Could you check a few things on this model? Use its own coordinates, in mm. Face numbers are marked on the shaded views. A direction names the side the tool comes from. Coordinates: 2 decimals unless noted, no trailing zeros. Write each loop counter-clockwise with the first axis right and the second up, starting at its lowest first coordinate (ties: lowest second). Pieces come first, ordered by that corner, then holes.
Item 1: Which directions (+Z, -Z, +X, -X, +Y, -Y) give clear straight access to the entire face, cutting with the end or side of a thin tool? Please do the marked faces 1, 2 and 3.
Item 2: For P1, Ø2, axis at y = -48, z = 42.5, coming from the -X side; P2, Ø12, axis at x = 35, z = 8, coming from the -Y side; P3, Ø3, axis at x = 10, z = 10, coming from the -Y side, each with a flat end and sliding along its axis, tell me the tip position at first contact or that it passes through.
Item 3: I want a section at B-B on x = -21. Please give me the cut outline in (y, z), then the cut area to 3 significant figures.
Item 4: I want a section at A-A on z = -2.5. Please give me the cut outline in (x, y).
Item 5: Thinking about a two-plate mould opening in X: for the marked faces 4, 5 and 6, which applies, +X half, -X half, draft (parallel to the pull), parting line (faces both ways), or undercut?
Item 6: I want a section at D-D on z = 5. Please give me the cut outline in (x, y), then the cut area to 3 significant figures.
Item 7: I want a section at C-C on z = 47.5. Please give me the cut outline in (x, y), then the cut area to 3 significant figures.
Item 8: If I drill on probe 1 along Z at (x, y) = (57, -18.5); probe 2 along Y at (x, z) = (-22, 42.5); probe 3 along Z at (x, y) = (4.5, -5), over which ranges is the centre line in solid material (lowest first)?
from build123d import *

# Parameters (mm, degrees)
F1_DEPTH = 60
F3_DEPTH = 60.001
F5_DEPTH = 100.001


with BuildPart() as f1:
    # F0 (on Front) → F1 (new body)
    with BuildSketch(Plane.XZ):
        Polygon((68.4196182877, 52.7130502019), (-31.5803817123, 52.7130502019), (-31.5803817123, -7.2869497981), (-11.5803817123, -7.2869497981), (-11.5803817123, 7.7130502019), (23.4196182877, 7.7130502019), (23.4196182877, -7.2869497981), (38.4196182877, -7.2869497981), (38.4196182877, 12.7130502019), (68.4196182877, 12.7130502019), align=None)
    extrude(amount=F1_DEPTH)

    # F2 (on face) → F3 (cut, through all)
    with BuildSketch(Plane(origin=(0, 0, -7.2869497981), x_dir=(1, 0, 0), z_dir=(0, 0, -1))):
        Polygon((68.4196182877, 60), (43.4196182877, 60), (68.4196182877, 35), align=None)
        Polygon((18.4196182877, 60), (-31.5803817123, 60), (-31.5803817123, 40), (-16.2213978636, 40), align=None)
    extrude(amount=-F3_DEPTH, mode=Mode.SUBTRACT)

    # F4 (on face) → F5 (cut, through all)
    with BuildSketch(Plane.YZ.offset(68.4196182877)):
        Polygon((-60, 42.7130502019), (-60, -7.2869497981), (-5, -7.2869497981), (-27, 12.7130502019), (-35, 12.7130502019), (-35, 19.9857774746), align=None)
        Polygon((-35, 12.7130502019), (-27, 12.7130502019), (-35, 19.9857774746), align=None)
    extrude(amount=-F5_DEPTH, mode=Mode.SUBTRACT)


solid = f1.part
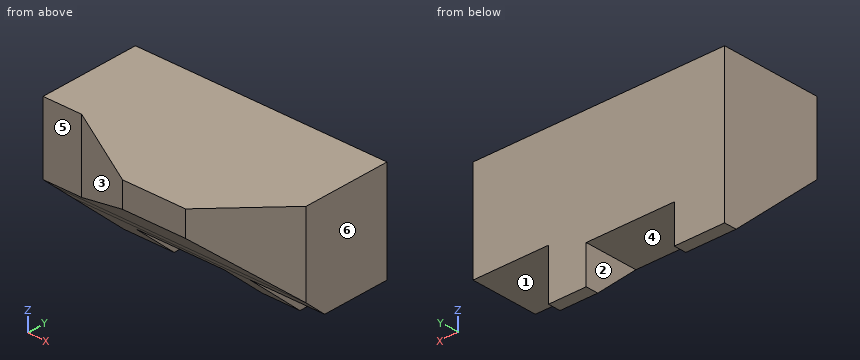
Response values:
1. face 1: -Z, +X, +Y, -Y
1. face 2: -Z, +Y, -Y
1. face 3: +Z, -Z, -X, -Y
2. P1: stops at x = -4.1
2. P2: stops at y = -28.42
2. P3: stops at y = -25.67
3. outline: (-40, 24.53) - (-5, -7.29) - (0, -7.29) - (0, 52.71) - (-40, 52.71) - close
3. area: 1,840 mm2
4. outline: (-31.58, -10.27) - (-11.58, -10.27) - (-11.58, 0) - (-31.58, 0) - close; (23.42, -10.27) - (38.42, -10.27) - (38.42, 0) - (23.42, 0) - close
5. face 4: undercut
5. face 5: draft
5. face 6: +X half
6. outline: (-31.58, -18.52) - (-11.58, -18.52) - (-11.58, 0) - (-31.58, 0) - close; (23.42, -18.52) - (38.42, -18.52) - (38.42, 0) - (23.42, 0) - close
6. area: 648 mm2
7. outline: (-31.58, -40) - (-16.22, -40) - (18.42, -60) - (43.42, -60) - (68.42, -35) - (68.42, 0) - (-31.58, 0) - close
7. area: 5,030 mm2
8. probe 1: z = 12.71 to 52.71
8. probe 2: y = -40 to 0
8. probe 3: z = 7.71 to 52.71
